For this review, take the finished solid that the model builds, in its own axes (mm). A direction names the side the tool comes from. Coordinates: 2 decimals unless noted, no trailing zeros. Write each loop counter-clockwise with the first axis right and the second up, starting at its lowest first coordinate (ties: lowest second). Pieces come first, ordered by that corner, then holes. Notation, with made-up numbers: (88.25, 51) - (105.25, 51) arc R26 ccw to (105.25, 88) - close; hole circle Ø4 at (70, 20.25). An arc over 180 degrees is marked (long way). Use one line per item in the form item = value. Start each with the question number.
1) For L1, parallel to X at y = -7, z = 3; L2, parallel to X at y = -6, z = 7.25; L3, parallel to Y at x = 12.5, z = 4.5, list the stretches that pass through material, from the lowest coordinate up. Write a range as from..to.
2) We need section B-B (z = 3.5). Give the boundary of the cut face in (x, y).
3) Tool access review of faces 4 (the flat face through (-13.17, 13.01, 9.01)), 5 (the flat face through (-12.45, 12.3, 3.94)), 6 (the flat face through (-50, -1, 3)): name each direction out of +Z, -Z, +X, -X, +Y, -Y from which nothing blocks a thin tool from reaching the whole face with its end or side.
4) We need section A-A (y = -3.5). Give the boundary of the cut face in (x, z), plus the area to 3 significant figures.
5) Mouldability with a two-part tool opening along X and no side actions: class faces 1 (the flat face through (13.17, -13.01, 9.01)), 2 (the flat face through (-1, 23, 0)), 3 (the cylindrical face through (-48.797, 0.7, 8.859)) as pulls with the +X half, pulls with the -X half, needs draft (parallel to the pull), parting line crosses it, or undercut.
6) Insertion check: P1, Ø3, axis at y = 34.5, z = 8, coming from the -X side. The pin has a flat end and moves straight along its axis. Give the tip position at first contact, or say it passes through.
```python
from build123d import *

# Parameters (mm, degrees)
F0_W     = 100
F0_H     = 100
F1_DEPTH = 10
F2_SIZE  = 2
F3_R     = 4


with BuildPart() as f1:
    # F0 (on Top) → F1 (new body)
    with BuildSketch(Plane.XY):
        Rectangle(F0_W, F0_H)
        Polygon((-17.5, 7.248737), (-7.248737, 17.5), (7.248737, 17.5), (17.5, 7.248737), (17.5, -7.248737), (7.248737, -17.5), (-7.248737, -17.5), (-17.5, -7.248737), align=None, mode=Mode.SUBTRACT)
    extrude(amount=F1_DEPTH)

    # F2
    f2_edges = [f1.edges().sort_by_distance(p)[0] for p in [
        (0, 17.5, 10),
        (12.374369, 12.374369, 10),
        (17.5, 0, 10),
        (12.374369, -12.374369, 10),
        (0, -17.5, 10),
        (-12.374369, -12.374369, 10),
        (-17.5, 0, 10),
        (-12.374369, 12.374369, 10),
    ]]
    chamfer(f2_edges, length=F2_SIZE)

    # F3
    f3_edges = [f1.edges().sort_by_distance(p)[0] for p in [
        (0, 50, 10),
        (50, 0, 10),
        (-50, 0, 10),
        (0, -50, 10),
    ]]
    fillet(f3_edges, radius=F3_R)


solid = f1.part
```
Determined:
q1.L1 = -50..-17.5, 17.5..50
q1.L2 = -49.8..-17.5, 17.5..49.8
q1.L3 = -50..-12.25, 12.25..50
q2.outline = (-50, -50) - (50, -50) - (50, 50) - (-50, 50) - close; hole (-17.5, -7.25) - (-7.25, -17.5) - (7.25, -17.5) - (17.5, -7.25) - (17.5, 7.25) - (7.25, 17.5) - (-7.25, 17.5) - (-17.5, 7.25) - close
q3.face_4 = +Z
q3.face_5 = +Z, -Z
q3.face_6 = +Z, -Z, -X, +Y, -Y
q4.outline = (-50, 0) - (-17.5, 0) - (-17.5, 8) - (-19.5, 10) - (-46, 10) arc R4 ccw to (-50, 6) - close; (17.5, 0) - (50, 0) - (50, 6) arc R4 ccw to (46, 10) - (19.5, 10) - (17.5, 8) - close
q4.area = 639 mm²
q5.face_1 = undercut
q5.face_2 = needs draft
q5.face_3 = pulls with the -X half
q6.P1 = -49.97
